Here's how the part is built. I have some questions about the finished solid (model axes, mm). Give positions to 0.01 mm unless a question says otherwise; leave off trailing zeros. Order: outer loops, then holes, each group sorted by start corner. A loop starts at its lowest first (then second) coordinate and runs counter-clockwise, first axis right, second up.
from build123d import *

# Parameters (mm, degrees)
F0_R     = 70
F0_R_2   = 3.5
F0_R_3   = 48
F1_DEPTH = 1.5875


with BuildPart() as f1:
    # F0 (on Top) → F1 (new body, symmetric)
    with BuildSketch(Plane.XY):
        Circle(F0_R)
        with Locations((0, -59.5)):
            Circle(F0_R_2, mode=Mode.SUBTRACT)
        with Locations((-59.5, 0)):
            Circle(F0_R_2, mode=Mode.SUBTRACT)
        Circle(F0_R_3, mode=Mode.SUBTRACT)
        with Locations((59.5, 0)):
            Circle(F0_R_2, mode=Mode.SUBTRACT)
        with Locations((0, 59.5)):
            Circle(F0_R_2, mode=Mode.SUBTRACT)
    extrude(amount=F1_DEPTH, both=True)


solid = f1.part
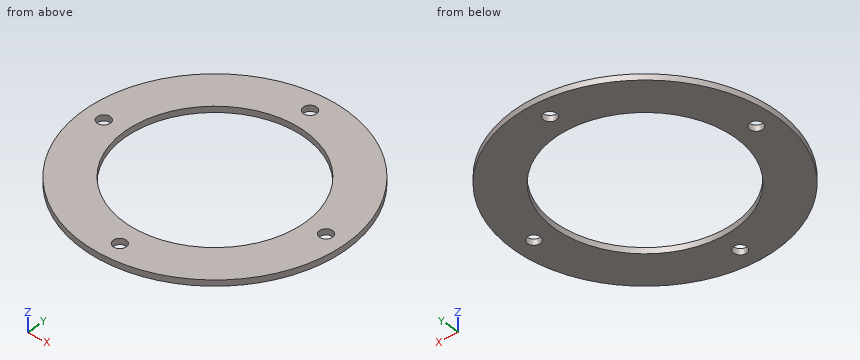
Q1. I need wall thicknesses on L1, parallel to Y at x = 0, z = 0.9; L2, parallel to Y at x = -58.5, z = 1; L3, parallel to Y at x = 4.5, z = -0.7. Which ranges of each line are inside material? Lowest first, please.
Filled sheet:
L1: y = -70 to -63, -56 to -48, 48 to 56, 63 to 70
L2: y = -38.44 to -3.35, 3.35 to 38.44
L3: y = -69.86 to -47.79, 47.79 to 69.86
Q2. If we section it at A-A on x = 0: List the corners of the cut face in (y, z) for me, plus the area to 4 significant figures.
Filled sheet:
outline: (-70, -1.59) - (-63, -1.59) - (-63, 1.59) - (-70, 1.59) - close; (-56, -1.59) - (-48, -1.59) - (-48, 1.59) - (-56, 1.59) - close; (48, -1.59) - (56, -1.59) - (56, 1.59) - (48, 1.59) - close; (63, -1.59) - (70, -1.59) - (70, 1.59) - (63, 1.59) - close
area: 95.25 mm2
Q3. If we section it at D-D on x = 34: List the corners of the cut face in (y, z) for me.
Filled sheet:
outline: (-61.19, -1.59) - (-33.88, -1.59) - (-33.88, 1.59) - (-61.19, 1.59) - close; (33.88, -1.59) - (61.19, -1.59) - (61.19, 1.59) - (33.88, 1.59) - close
Q4. If we section it at C-C on z = 0.95: List the corners of the cut face in (x, y) for me, plus the area to 3 significant figures.
Filled sheet:
outline: circle Ø140 at (0, 0); hole circle Ø7 at (-59.5, 0); hole circle Ø96 at (0, 0); hole circle Ø7 at (0, -59.5); hole circle Ø7 at (0, 59.5); hole circle Ø7 at (59.5, 0)
area: 8,000 mm2
Q5. If we section it at B-B on y = -59.5: List the corners of the cut face in (x, z) for me.
Filled sheet:
outline: (-36.87, -1.59) - (-3.5, -1.59) - (-3.5, 1.59) - (-36.87, 1.59) - close; (3.5, -1.59) - (36.87, -1.59) - (36.87, 1.59) - (3.5, 1.59) - close
Q6. I'm going to push a flat-ended pin straight in: P1, Ø1.5, axis at y = -2.5, z = -0.5, coming from the +X side. Where does the tip first touch, or does it pass through?
Filled sheet:
P1: stops at x = 69.98
